The model under review builds one solid part; all positions refer to its coordinate system, in mm. A direction names the side the tool comes from. Coordinates: 2 decimals unless noted, no trailing zeros. Write each loop counter-clockwise with the first axis right and the second up, starting at its lowest first coordinate (ties: lowest second). Pieces come first, ordered by that corner, then holes. Notation, with made-up numbers: (35.25, -5.5) -> (70.25, -5.5) arc R33 cw to (70.25, 30.5) -> close; hole circle Ø3 at (33, 43). An arc over 180 degrees is marked (long way). Write each question's results on one line, items separated by ' | '.
```python
from build123d import *


with BuildPart() as part:
    # Sketch1 → Revolve1 (revolve)
    with BuildSketch(Plane(origin=(0, 0, 0), x_dir=(1, 0, 0), z_dir=(0, 1, 0))):
        with BuildLine():
            Line((25.4, 0), (19.05, 0))
            Line((19.05, 0), (19.05, -19.05))
            Line((19.05, -19.05), (21.535759249, -19.05))
            Line((21.535759249, -19.05), (22.225, -17.8562))
            Line((22.225, -17.8562), (22.225, -3.675))
            ThreePointArc((22.225, -3.675), (22.371446609, -3.321446609), (22.725, -3.175))
            Line((22.725, -3.175), (25.4, -3.175))
            Line((25.4, -3.175), (25.4, 0))
        make_face()
    revolve(axis=Axis((0, 0, 0), (0, 0, 1)))


solid = part.part
```
Q1. Add section C-C (z = 1.5). Write out the cut boundary in (x, y), plus the area to 3 significant figures.
Solution:
outline: circle Ø50.8 at (0, 0); hole circle Ø38.1 at (0, 0) | area: 887 mm²
Q2. Draft analysis for pull direction Y (two halves, no side actions). For faces 1 (the flat face through (8.08, -17.45, 19.05)), 2 (the cylindrical face through (-15.12, -11.59, 9.66)), 3 (the cylindrical face through (-5.506, -24.796, 1.565)), state which applies: pulls with the +Y half, pulls with the -Y half, needs draft (parallel to the pull), parting line crosses it, or undercut.
Solution:
face 1: needs draft | face 2: undercut | face 3: parting line crosses it
Q3. Add section D-D (z = 9). Write out the cut boundary in (x, y) (3 decimals).
Solution:
outline: circle Ø44.45 at (0, 0); hole circle Ø38.1 at (0, 0)
Q4. Machinability: for faces 4 (the cylindrical face through (21.199, 6.676, 10.666)), 5 (the flat face through (4, 19, 0)), which of the approach directions +Z, -Z, +X, -X, +Y, -Y give a long, thin tool a straight path to every point of the face, cutting with its end or side? Answer none if there is none.
Solution:
face 4: +Z | face 5: -Z, +X, -X, +Y, -Y
Q5. Add section A-A (x = 0). Write out the cut boundary in (y, z) (3 decimals).
Solution:
outline: (-25.4, 0) -> (-19.05, 0) -> (-19.05, 19.05) -> (-21.536, 19.05) -> (-22.225, 17.856) -> (-22.225, 3.675) arc R0.5 cw to (-22.725, 3.175) -> (-25.4, 3.175) -> close; (19.05, 0) -> (25.4, 0) -> (25.4, 3.175) -> (22.725, 3.175) arc R0.5 cw to (22.225, 3.675) -> (22.225, 17.856) -> (21.536, 19.05) -> (19.05, 19.05) -> close
Q6. For line 1 (Y direction, x = 0, z = 6) (3 decimals); line 2 (Z direction, x = -12, y = -21.5) (3 decimals); line 3 (Y direction, x = 8, z = 3), list the stretches that pass through material, from the lowest coordinate up. Write a range as from..to.
Solution:
line 1: -22.225..-19.05, 19.05..22.225 | line 2: 0..3.175 | line 3: -24.11..-17.29, 17.29..24.11
Q7. Clearance check with flat-ended pins moving along their axes: P1, Ø6, axis at x = -14.5, z = 14.5, coming from the +Y side; P2, Ø1, axis at y = 18, z = 7.5, coming from the -X side; P3, Ø2, axis at x = 17, z = 10, coming from the +Y side. State where each tip first meets the part, or that it passes through.
Solution:
P1: y = 19.02 | P2: x = -13.7 | P3: y = 15.43
